The figure shows three views and two pictorial views of one solid part (mm, origin at its lowest corner). Answer the questions. Give positions to 0.01 mm unless a question says otherwise; leave off trailing zeros. Loops run counter-clockwise (first coordinate to the right, second up) from the corner with the lowest first, then second, coordinate; pieces in that order, holes last.
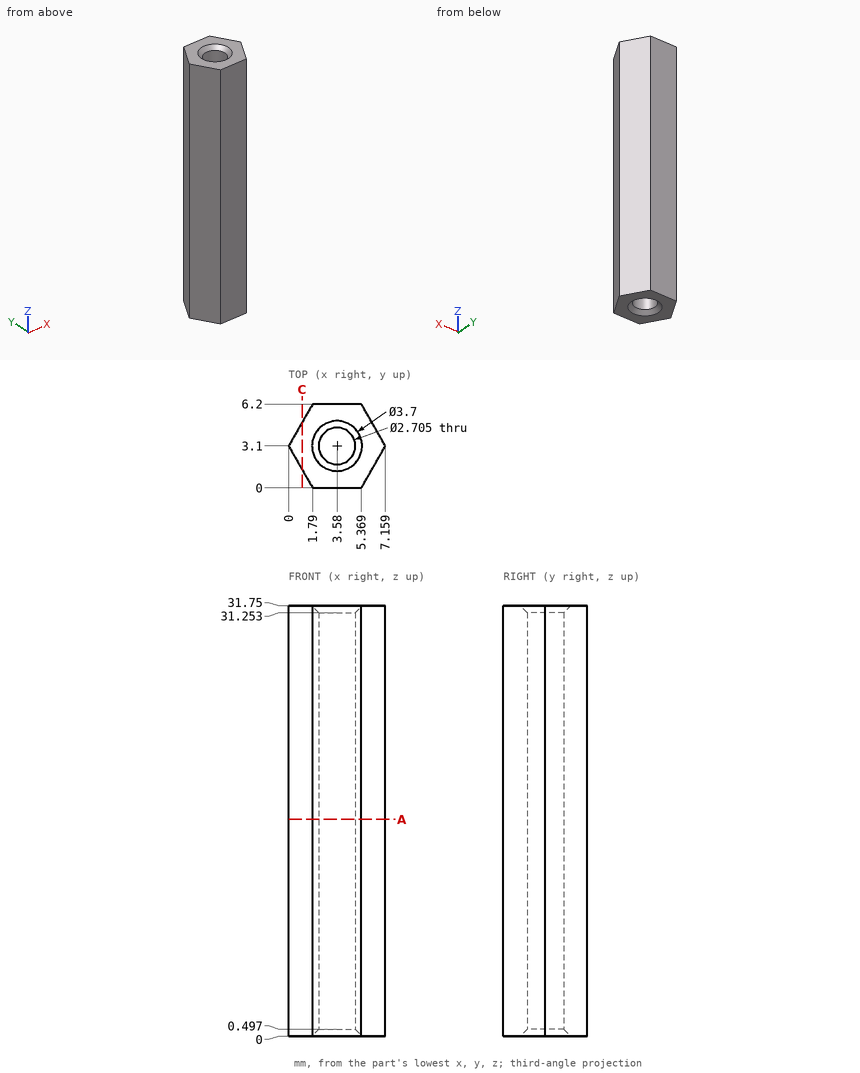
Q1. Given pin 1 (3 mm diameter, centred on y = 3.5, z = 7, fed in from -X); pin 2 (2 mm diameter, centred on x = 3.58, y = 3.1, fed in from -Z), each flat-ended and moving along its own axis, determine where each tip first touches the part or whether it passes through.
Q2. Consider line 1 along Y through (x, z) = (4.25, 22) (1 decimal); line 2 along Y through (x, z) = (3.25, 9.5); line 3 along X through (y, z) = (3.25, 18) (1 decimal). Determine where each line is inside the solid, lowest interval first.
Q3. Section C-C on x = 1 is taken. Give the vertices of the cut face in (y, z), plus the area to 3 significant figures.
Q4. Section A-A on z = 16 is taken. Give the vertices of the cut face in (x, y) (1 decimal).
Check result:
1. pin 1: stops at x = 0
1. pin 2: passes through
2. line 1: y = 0 to 1.9, 4.3 to 6.2
2. line 2: y = 0 to 1.79, 4.41 to 6.2
2. line 3: x = 0.1 to 2.2, 4.9 to 7.1
3. outline: (1.37, 0) - (4.83, 0) - (4.83, 31.75) - (1.37, 31.75) - close
3. area: 110 mm2
4. outline: (0, 3.1) - (1.8, 0) - (5.4, 0) - (7.2, 3.1) - (5.4, 6.2) - (1.8, 6.2) - close; hole circle Ø2.7 at (3.6, 3.1)
